Check sheet for the modelled part. Datum: model origin and axes. Units: mm. A direction names the side the tool comes from. Give positions to 0.01 mm unless a question says otherwise; leave off trailing zeros. Order: outer loops, then holes, each group sorted by start corner. A loop starts at its lowest first (then second) coordinate and runs counter-clockwise, first axis right, second up. Notation, with made-up numbers: (78.25, 27) - (85.25, 27) arc R18 cw to (85.25, 44) - close; hole circle Ø10 at (14.5, -26.75). An arc over 180 degrees is marked (long way). Answer in a Markdown table with one row per item.
from build123d import *

# Parameters (mm, degrees)
BOSS_EXTRUDE1_DEPTH = 9
CUT_EXTRUDE2_REACH  = 97.631
SKETCH5_W           = 20
SKETCH5_H           = 32
SKETCH5_W_2         = 7.75
CUT_EXTRUDE3_DEPTH  = 10
FILLET1_R           = 5
CUT_EXTRUDE4_DEPTH  = 4
CHAMFER1_SIZE       = 9
CHAMFER1_SIZE_2     = 4.196768923
FILLET2_R           = 10
CUT_EXTRUDE5_REACH  = 97.631
SKETCH7_W           = 5
SKETCH7_H           = 33.085129134
SKETCH7_H_2         = 33.745309592


with BuildPart() as part:
    # Sketch1 → Boss-Extrude1 (new body)
    with BuildSketch(Plane(origin=(0, 0, 0), x_dir=(1, 0, 0), z_dir=(0, 1, 0))):
        Polygon((0, 0), (0, 58), (75.5, 58), (75.5, 0), (37.75, 17.603114095), align=None)
    extrude(amount=BOSS_EXTRUDE1_DEPTH)

    # Sketch4 → Cut-Extrude2 (cut, up to next)
    with BuildSketch(Plane(origin=(0, 9, 0), x_dir=(1, 0, 0), z_dir=(0, 1, 0)), mode=Mode.PRIVATE) as cut_extrude2_sk1:
        with BuildLine():
            Line((19.25, 51), (19.25, 26))
            ThreePointArc((19.25, 26), (17.75, 24.5), (16.25, 26))
            Line((16.25, 26), (16.25, 51))
            ThreePointArc((16.25, 51), (17.75, 52.5), (19.25, 51))
        make_face()
    cut_extrude2_tool1 = extrude(cut_extrude2_sk1.sketch, amount=-CUT_EXTRUDE2_REACH, mode=Mode.PRIVATE) & part.part
    # Sketch4 → Cut-Extrude2 (cut, up to next)
    with BuildSketch(Plane(origin=(0, 9, 0), x_dir=(1, 0, 0), z_dir=(0, 1, 0)), mode=Mode.PRIVATE) as cut_extrude2_sk2:
        with BuildLine():
            Line((59.25, 51), (59.25, 26))
            ThreePointArc((59.25, 26), (57.75, 24.5), (56.25, 26))
            Line((56.25, 26), (56.25, 51))
            ThreePointArc((56.25, 51), (57.75, 52.5), (59.25, 51))
        make_face()
    cut_extrude2_tool2 = extrude(cut_extrude2_sk2.sketch, amount=-CUT_EXTRUDE2_REACH, mode=Mode.PRIVATE) & part.part
    add(cut_extrude2_tool1.solids().sort_by_distance((17.75, 9, -38.5))[0], mode=Mode.SUBTRACT)
    add(cut_extrude2_tool2.solids().sort_by_distance((57.75, 9, -38.5))[0], mode=Mode.SUBTRACT)

    # Sketch5 → Cut-Extrude3 (cut)
    with BuildSketch(Plane(origin=(0, 9, 0), x_dir=(1, 0, 0), z_dir=(0, 1, 0))):
        with Locations((37.75, 42)):
            Rectangle(SKETCH5_W, SKETCH5_H)
        with Locations((71.625, 42)):
            Rectangle(SKETCH5_W_2, SKETCH5_H)
        with Locations((3.875, 42)):
            Rectangle(SKETCH5_W_2, SKETCH5_H)
    extrude(amount=-CUT_EXTRUDE3_DEPTH, mode=Mode.SUBTRACT)

    # Fillet1
    fillet1_edges = [part.edges().sort_by_distance(p)[0] for p in [
        (27.75, 4.5, -26),
        (47.75, 4.5, -26),
        (7.75, 4.5, -26),
        (67.75, 4.5, -26),
    ]]
    fillet(fillet1_edges, radius=FILLET1_R)

    # Sketch6 → Cut-Extrude4 (cut)
    with BuildSketch(Plane(origin=(0, 9, 0), x_dir=(1, 0, 0), z_dir=(0, 1, 0))):
        with BuildLine():
            Line((20.55, 51), (20.55, 26))
            ThreePointArc((20.55, 26), (17.75, 23.2), (14.95, 26))
            Line((14.95, 26), (14.95, 51))
            ThreePointArc((14.95, 51), (17.75, 53.8), (20.55, 51))
        make_face()
        with BuildLine():
            Line((60.55, 51), (60.55, 26))
            ThreePointArc((60.55, 26), (57.75, 23.2), (54.95, 26))
            Line((54.95, 26), (54.95, 51))
            ThreePointArc((54.95, 51), (57.75, 53.8), (60.55, 51))
        make_face()
    extrude(amount=-CUT_EXTRUDE4_DEPTH, mode=Mode.SUBTRACT)

    # Chamfer1
    # the kernel refuses this chamfer: 9, 4.196768923 mm, written as the material it takes off along each edge
    with BuildSketch(Plane(origin=(96.633991212, 9, 9.85494195), x_dir=(-0.006893395832057369, -0.9998669641130703, 0.014782935067658582), z_dir=(-0.9063077870366479, 0, -0.42261826174070394))) as chamfer1_piece_1_section:
        Polygon((CHAMFER1_SIZE * 0.999866964113, -CHAMFER1_SIZE * 0.0163111641311), (-CHAMFER1_SIZE_2 * 0.0163111641326, -CHAMFER1_SIZE_2 * 0.999866964207), (0, 0), align=None)
    chamfer1_piece_1 = extrude(amount=88.290074926, mode=Mode.PRIVATE)
    chamfer1_piece_1 = split(chamfer1_piece_1, bisect_by=Plane(origin=(57.902621458, 5.937801532, -27.000435813), z_dir=(0.42261826174070394, 0, 0.9063077870366479)), keep=Keep.TOP, mode=Mode.PRIVATE)
    add(chamfer1_piece_1, mode=Mode.SUBTRACT)
    with BuildSketch(Plane(origin=(58.883991212, 9, -27.458056045), x_dir=(0.006893395832057004, -0.9998669641130703, 0.014782935067657803), z_dir=(-0.9063077870366479, 0, 0.42261826174070394))) as chamfer1_piece_2_section:
        Polygon((CHAMFER1_SIZE * 0.999866964113, -CHAMFER1_SIZE * 0.0163111641311), (-CHAMFER1_SIZE_2 * 0.0163111641326, -CHAMFER1_SIZE_2 * 0.999866964207), (0, 0), align=None)
    chamfer1_piece_2 = extrude(amount=88.290074926, mode=Mode.PRIVATE)
    chamfer1_piece_2 = split(chamfer1_piece_2, bisect_by=Plane(origin=(17.597378542, 5.937801532, -27.000435813), z_dir=(-0.42261826174070394, 0, 0.9063077870366479)), keep=Keep.TOP, mode=Mode.PRIVATE)
    add(chamfer1_piece_2, mode=Mode.SUBTRACT)
    with BuildSketch(Plane(origin=(96.633991212, 9, 9.85494195), x_dir=(-0.006893395832057369, -0.9998669641130703, 0.014782935067658582), z_dir=(-0.9063077870366479, 0, -0.42261826174070394))) as chamfer1_piece_3a_section:
        Polygon((CHAMFER1_SIZE * 0.999866964113, -CHAMFER1_SIZE * 0.0163111641311), (-CHAMFER1_SIZE_2 * 0.0163111641326, -CHAMFER1_SIZE_2 * 0.999866964207), (0, 0), align=None)
    chamfer1_piece_3a = extrude(amount=88.290074926, mode=Mode.PRIVATE)
    chamfer1_piece_3a = split(chamfer1_piece_3a, bisect_by=Plane(origin=(32.238129018, 6.0031385, -15.032886446), z_dir=(-0.42261826174070394, 0, -0.9063077870366479)), keep=Keep.TOP, mode=Mode.PRIVATE)
    with BuildSketch(Plane(origin=(58.883991212, 9, -27.458056045), x_dir=(0.006893395832057004, -0.9998669641130703, 0.014782935067657803), z_dir=(-0.9063077870366479, 0, 0.42261826174070394))) as chamfer1_piece_3b_section:
        Polygon((CHAMFER1_SIZE * 0.999866964113, -CHAMFER1_SIZE * 0.0163111641311), (-CHAMFER1_SIZE_2 * 0.0163111641326, -CHAMFER1_SIZE_2 * 0.999866964207), (0, 0), align=None)
    chamfer1_piece_3b = extrude(amount=88.290074926, mode=Mode.PRIVATE)
    chamfer1_piece_3b = split(chamfer1_piece_3b, bisect_by=Plane(origin=(43.261870982, 6.0031385, -15.032886446), z_dir=(0.42261826174070394, 0, -0.9063077870366479)), keep=Keep.TOP, mode=Mode.PRIVATE)
    chamfer1_piece_3 = chamfer1_piece_3a & chamfer1_piece_3b
    add(chamfer1_piece_3, mode=Mode.SUBTRACT)

    # Fillet2
    fillet2_edges = [part.edges().sort_by_distance(p)[0] for p in [
        (37.75, 4.5, -19.918425176),
    ]]
    fillet(fillet2_edges, radius=FILLET2_R)

    # Sketch7 → Cut-Extrude5 (cut, up to next)
    with BuildSketch(Plane(origin=(0, 9, 0), x_dir=(1, 0, 0), z_dir=(0, 1, 0)), mode=Mode.PRIVATE) as cut_extrude5_sk1:
        with Locations((2.5, 16.542564567)):
            Rectangle(SKETCH7_W, SKETCH7_H)
    cut_extrude5_tool1 = extrude(cut_extrude5_sk1.sketch, amount=-CUT_EXTRUDE5_REACH, mode=Mode.PRIVATE) & part.part
    # Sketch7 → Cut-Extrude5 (cut, up to next)
    with BuildSketch(Plane(origin=(0, 9, 0), x_dir=(1, 0, 0), z_dir=(0, 1, 0)), mode=Mode.PRIVATE) as cut_extrude5_sk2:
        with Locations((73, 16.872654796)):
            Rectangle(SKETCH7_W, SKETCH7_H_2)
    cut_extrude5_tool2 = extrude(cut_extrude5_sk2.sketch, amount=-CUT_EXTRUDE5_REACH, mode=Mode.PRIVATE) & part.part
    add(cut_extrude5_tool1.solids().sort_by_distance((2.5, 9, -16.542565))[0], mode=Mode.SUBTRACT)
    add(cut_extrude5_tool2.solids().sort_by_distance((73, 9, -16.872655))[0], mode=Mode.SUBTRACT)


solid = part.part
(1) Cross-section at B-B, the plane x = 57.75. Record the cut outline in (y, z), then the cut area to 3 significant figures.
Geometry says:
| item | result |
|---|---|
| outline | (0, -58) - (9, -58) - (9, -53.8) - (5, -53.8) - (5, -52.5) - (0, -52.5) - close; (0, -24.5) - (5, -24.5) - (5, -23.2) - (9, -23.2) - (9, -12.91) - (0, -8.28) - close |
| area | 164 mm² |
(2) Thickness scan on L1, parallel to X at y = 4.75, z = -36; L2, parallel to X at y = 7, z = -33; L3, parallel to X at y = 8, z = -55. Record the ranges inside material, lowest first.
Geometry says:
| item | result |
|---|---|
| L1 | 7.75 to 16.25, 19.25 to 27.75, 47.75 to 56.25, 59.25 to 67.75 |
| L2 | 7.75 to 14.95, 20.55 to 27.75, 47.75 to 54.95, 60.55 to 67.75 |
| L3 | 7.75 to 27.75, 47.75 to 67.75 |
(3) Gauge pin test, flat ends, axial feed: P1, Ø2, axis at y = 7, z = -33.5, coming from the +X side; P2, Ø3, axis at x = 57.5, z = -32.5, coming from the +Y side; P3, Ø2, axis at y = 7.5, z = -37, coming from the -X side. Record the tip position at first contact, or that the pin passes through.
Geometry says:
| item | result |
|---|---|
| P1 | x = 67.75 |
| P2 | y = 5 |
| P3 | x = 7.75 |
(4) Access from +Z, -Z, +X, -X, +Y, -Y to the whole of each face (thin tool, end or side, straight path). Record for faces 1 (the flat face through (7.75, 5, -44)), 2 (the cylindrical face through (17.8, 7, -23.2)), 3 (the flat face through (67.75, 5, -44)), 4 (the cylindrical face through (57.7, 2.5, -52.5)), 5 (the flat face through (27.75, 5, -44)).
Geometry says:
| item | result |
|---|---|
| face 1 | -Z, -X, +Y, -Y |
| face 2 | +Y |
| face 3 | -Z, +X, +Y, -Y |
| face 4 | +Y, -Y |
| face 5 | -Z, +Y, -Y |
(5) Cross-section at D-D, the plane z = -29. Record the cut outline in (x, y).
Geometry says:
| item | result |
|---|---|
| outline | (7.33, 0) - (16.25, 0) - (16.25, 5) - (14.95, 5) - (14.95, 9) - (7.33, 9) - close; (19.25, 0) - (28.17, 0) - (28.17, 9) - (20.55, 9) - (20.55, 5) - (19.25, 5) - close; (47.33, 0) - (56.25, 0) - (56.25, 5) - (54.95, 5) - (54.95, 9) - (47.33, 9) - close; (59.25, 0) - (68.17, 0) - (68.17, 9) - (60.55, 9) - (60.55, 5) - (59.25, 5) - close |
(6) Mould release check, pull along Z, two halves, no side actions. Record for faces 6 (the flat face through (19.687, 4.437, -11.463)), 7 (the cylindrical face through (57.8, 2.5, -24.5)), 8 (the flat face through (58, 4, -58)), 9 (the flat face through (5, 5, -14)): pulls with the +Z half, pulls with the -Z half, needs draft (parallel to the pull), parting line crosses it, or undercut.
Geometry says:
| item | result |
|---|---|
| face 6 | pulls with the +Z half |
| face 7 | undercut |
| face 8 | pulls with the -Z half |
| face 9 | needs draft |
(7) Cross-section at C-C, the plane y = 4.25. Give the number of separate pieces and of enclosed holes in the cut face, then the cut area to 3 significant figures.
Geometry says:
| item | result |
|---|---|
| separate pieces | 1 |
| enclosed holes | 2 |
| area | 2,050 mm² |
(8) Cross-section at A-A, the plane z = -37. Record the cut outline in (x, y), then the cut area to 3 significant figures.
Geometry says:
| item | result |
|---|---|
| outline | (7.75, 0) - (16.25, 0) - (16.25, 5) - (14.95, 5) - (14.95, 9) - (7.75, 9) - close; (19.25, 0) - (27.75, 0) - (27.75, 9) - (20.55, 9) - (20.55, 5) - (19.25, 5) - close; (47.75, 0) - (56.25, 0) - (56.25, 5) - (54.95, 5) - (54.95, 9) - (47.75, 9) - close; (59.25, 0) - (67.75, 0) - (67.75, 9) - (60.55, 9) - (60.55, 5) - (59.25, 5) - close |
| area | 285 mm² |
